The drawing under review shows one solid part. Ordinate dimensions are in mm from its lowest x, y, z. A direction names the side the tool comes from. Round coordinates to 2 decimals unless told otherwise and drop trailing zeros. Order: outer loops, then holes, each group sorted by start corner. A loop starts at its lowest first (then second) coordinate and runs counter-clockwise, first axis right, second up.
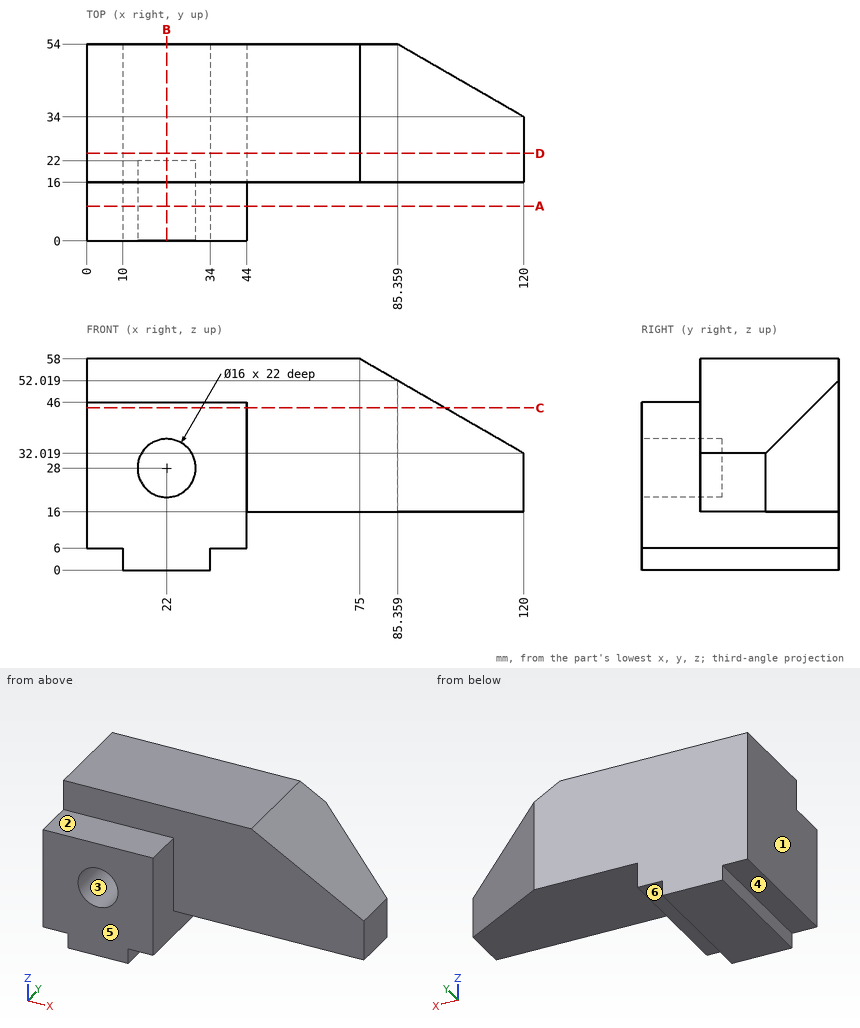
Q1. Tool access review of the marked faces 4, 5 and 6: name each direction out of +Z, -Z, +X, -X, +Y, -Y from which nothing blocks a thin tool from reaching the whole face with its end or side.
Q2. Take a section at A-A, the plane y = 9.5. State the section outline as (x, z) points, plus the area to 3 significant figures.
Q3. Take a section at B-B, the plane x = 22. State the section outline as (y, z) points.
Q4. Wall thickness on line 1 (Z direction, x = 22, y = 13.5); line 2 (Z direction, x = 22, y = 17); line 3 (X direction, y = 39, z = 12.5): over which ranges is each line inside the solid? List them lowest first.
Q5. Clearance check with flat-ended pins moving along their axes: pin 1 (1 mm diameter, centred on x = 79.5, y = 15, fed in from -Z); pin 2 (4 mm diameter, centred on y = 18, z = 7, fed in from +X); pin 3 (12.5 mm diameter, centred on x = 60, z = 47.5, fed in from -Y); pin 4 (1.8 mm diameter, centred on y = 28, z = 2.5, fed in from +X). State where each tip first meets the part, or that it passes through.
Q6. Take a section at D-D, the plane y = 24. State the section outline as (x, z) points.
Q7. Mouldability with a two-part tool opening along X and no side actions: class the marked faces 1, 2 and 3 as +X half, -X half, draft (parallel to the pull), parting line (faces both ways), or undercut.
Q8. Take a section at C-C, the plane z = 44.5. State the section outline as (x, y) points.
Working result:
1. face 4: -Z, -X, +Y, -Y
1. face 5: +Z, -Z, +X, -X, -Y
1. face 6: -Z, +X, +Y, -Y
2. outline: (0, 6) - (10, 6) - (10, 0) - (34, 0) - (34, 6) - (44, 6) - (44, 46) - (0, 46) - close; hole circle Ø16 at (22, 28)
2. area: 1,700 mm2
3. outline: (0, 0) - (54, 0) - (54, 58) - (16, 58) - (16, 46) - (0, 46) - (0, 36) - (22, 36) - (22, 20) - (0, 20) - close
4. line 1: z = 0 to 20, 36 to 46
4. line 2: z = 0 to 20, 36 to 58
4. line 3: x = 0 to 44
5. pin 1: passes through
5. pin 2: stops at x = 44
5. pin 3: stops at y = 16
5. pin 4: stops at x = 34
6. outline: (0, 6) - (10, 6) - (10, 0) - (34, 0) - (34, 6) - (44, 6) - (44, 16) - (120, 16) - (120, 32.02) - (75, 58) - (0, 58) - close
7. face 1: -X half
7. face 2: draft
7. face 3: undercut
8. outline: (0, 0) - (44, 0) - (44, 16) - (98.38, 16) - (98.38, 46.48) - (85.36, 54) - (0, 54) - close
